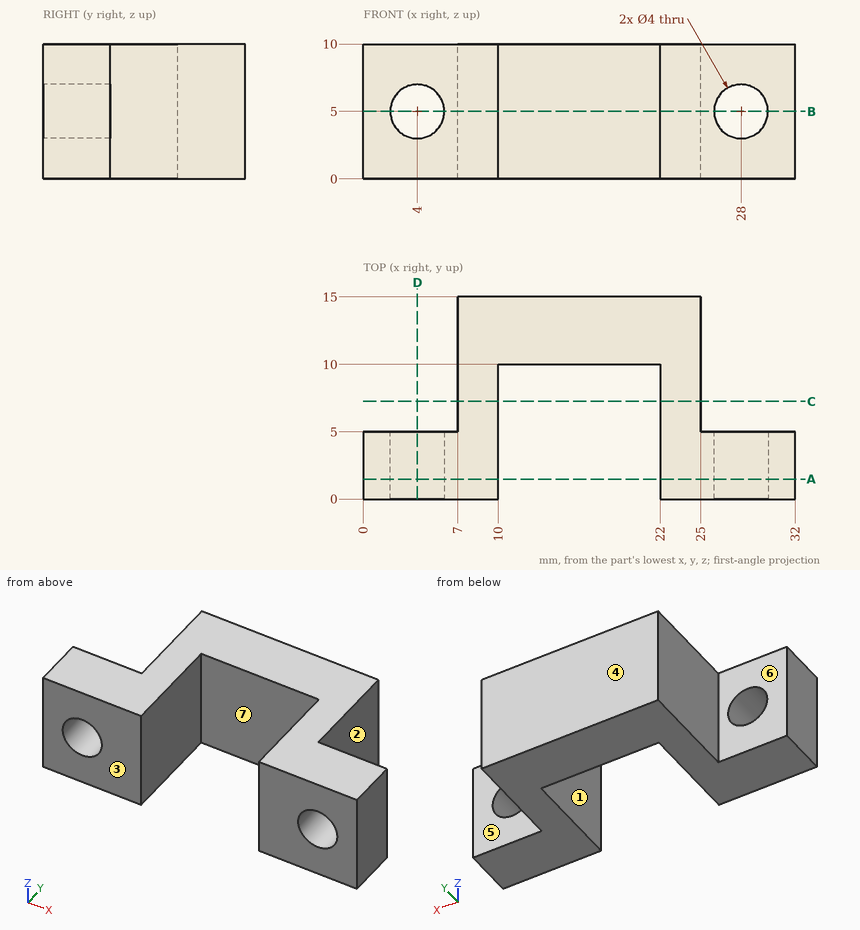
Part print with two shaded views. Sizes in mm from the minimum x, y, z corner. A direction names the side the tool comes from. Coordinates: 2 decimals unless noted, no trailing zeros. Order: outer loops, then holes, each group sorted by start corner. A loop starts at its lowest first (then second) coordinate and runs counter-clockwise, first axis right, second up. Notation, with made-up numbers: (53.25, -17.75) - (81.25, -17.75) arc R37 cw to (81.25, 19.25) - close; hole circle Ø5 at (39.25, 74). An arc over 180 degrees is marked (long way). Answer in a Markdown table with one row per item.
1. Slice it at A-A, the plane y = 1.5. List the corners of the cut face in (x, z), then the cut area to 3 significant figures.
Answer:
| item | result |
|---|---|
| outline | (0, 0) - (10, 0) - (10, 10) - (0, 10) - close; (22, 0) - (32, 0) - (32, 10) - (22, 10) - close; hole circle Ø4 at (4, 5); hole circle Ø4 at (28, 5) |
| area | 175 mm² |
2. Slice it at D-D, the plane x = 4. List the corners of the cut face in (y, z), then the cut area to 3 significant figures.
Answer:
| item | result |
|---|---|
| outline | (0, 0) - (5, 0) - (5, 3) - (0, 3) - close; (0, 7) - (5, 7) - (5, 10) - (0, 10) - close |
| area | 30.0 mm² |
3. Drill centre lines: L1, parallel to X at y = 1.95, z = 5; L2, parallel to Z at x = 4, y = 1.1; L3, parallel to X at y = 9.5, z = 6.25. Where is each one in solid material? Low to high. Write a range as from..to.
Answer:
| item | result |
|---|---|
| L1 | 0..2, 6..10, 22..26, 30..32 |
| L2 | 0..3, 7..10 |
| L3 | 7..10, 22..25 |
4. Flat gauge pins, fed straight in: P1, Ø3.5, axis at x = 28, z = 2.5, coming from the +Y side; P2, Ø5, axis at y = 11.5, z = 3.5, coming from the +X side; P3, Ø3, axis at y = 5.5, z = 3, coming from the +X side; P4, Ø1, axis at y = 13, z = 6.5, coming from the -X side. Where does each tip first touch, or does it go through?
Answer:
| item | result |
|---|---|
| P1 | y = 5 |
| P2 | x = 25 |
| P3 | x = 32 |
| P4 | x = 7 |
5. Slice it at C-C, the plane y = 7.25. List the corners of the cut face in (x, z), then the cut area to 3 significant figures.
Answer:
| item | result |
|---|---|
| outline | (7, 0) - (10, 0) - (10, 10) - (7, 10) - close; (22, 0) - (25, 0) - (25, 10) - (22, 10) - close |
| area | 60.0 mm² |
6. 3-axis set-ups, long thin cutter, end or side, ignore diameter. For the marked faces 4, 5, 6 and 7: which of +Z, -Z, +X, -X, +Y, -Y reach the whole face in a straight line?
Answer:
| item | result |
|---|---|
| face 4 | +Z, -Z, +X, -X, +Y |
| face 5 | +Z, -Z, +X, +Y |
| face 6 | +Z, -Z, -X, +Y |
| face 7 | +Z, -Z, -Y |
7. Pull direction X, two halves, no side cores. Call the marked faces 1, 2 and 3: +X half, -X half, draft (parallel to the pull), parting line (faces both ways), or undercut.
Answer:
| item | result |
|---|---|
| face 1 | undercut |
| face 2 | +X half |
| face 3 | draft |
8. Slice it at B-B, the plane z = 5. List the corners of the cut face in (x, y), then the cut area to 3 significant figures.
Answer:
| item | result |
|---|---|
| outline | (0, 0) - (2, 0) - (2, 5) - (0, 5) - close; (6, 0) - (10, 0) - (10, 10) - (22, 10) - (22, 0) - (26, 0) - (26, 5) - (25, 5) - (25, 15) - (7, 15) - (7, 5) - (6, 5) - close; (30, 0) - (32, 0) - (32, 5) - (30, 5) - close |
| area | 180 mm² |
